Geometry: final body of the model. Coordinates: model frame, mm. A direction names the side the tool comes from. Give positions to 0.01 mm unless a question says otherwise; leave off trailing zeros. Write each loop counter-clockwise with the first axis right and the second up, starting at its lowest first coordinate (ties: lowest second). Pieces come first, ordered by that corner, then holes. Notation, with made-up numbers: (-37, -13) -> (5, -13) arc R23 ccw to (5, 22) -> close; hole circle Ø5 at (82, 71). An arc over 180 degrees is marked (long way). Answer in a Markdown table with one row per item. Add a question column.
Item 1: Material intervals for probe 1 along Y at (x, z) = (48, 13.25); probe 2 along Y at (x, z) = (31, 8.5); probe 3 along X at (y, z) = (18, 4.75), sorted ascending. Write a range as from..to.
Item 2: Section query A-A on x = 51. Output: boundary loops of the cut face in (y, z).
Item 3: Section query D-D on x = -29. Output: boundary loops of the cut face in (y, z), plus the area to 3 significant figures.
Item 4: Section query C-C on y = 31.5. Output: boundary loops of the cut face in (x, z).
Item 5: First-contact query: P1, Ø1.6, axis at x = -0.5, z = 11, coming from the +Y side. Flat tip, straight axial feed; report the tip coordinate or a pass-through.
Item 6: Access query for faces 1 (the cylindrical face through (-8.61, -38.76, 9.86)), 2 (the flat face through (-2.813, 48.08, 11.511)), 3 (the flat face through (63.72, -3.73, 12.2)). Directions: +Z, -Z, +X, -X, +Y, -Y. A direction counts if a zero-diameter tool reaches every point of the face in a straight line with its end or side. Return the directions, or none.
Item 7: Section query B-B on y = 0. Output: boundary loops of the cut face in (x, z).
Item 8: Draft query along Z for faces 4 (the cylindrical face through (-84.53, 46.98, 9.86)), 5 (the flat face through (63.72, 3.73, 7.8)), 6 (the flat face through (40, 1, 20)). Return one class per face: +Z half, -Z half, draft (parallel to the pull), parting line (faces both ways), or undercut.
```python
from build123d import *

# Parameters (mm, degrees)
SKETCH1_R               = 39.705202959
BOSS_EXTRUDE1_DEPTH     = 20
CUT_EXTRUDE1_DEPTH      = 5
CUT_EXTRUDE1_DRAFT      = -24
CUT_EXTRUDE2_REACH      = 184.868
CUT_EXTRUDE2_END_RADIUS = 39.705202959


with BuildPart() as part:
    # Sketch1 → Boss-Extrude1 (new body)
    with BuildSketch(Plane.XY):
        with BuildLine():
            Line((77.380717994, -49.989899132), (-77.380717994, -49.989899132))
            ThreePointArc((-77.380717994, -49.989899132), (-84.451785806, -47.060966943), (-87.380717994, -39.989899132))
            Line((-87.380717994, -39.989899132), (-87.380717994, 39.989899132))
            ThreePointArc((-87.380717994, 39.989899132), (-84.451785806, 47.060966943), (-77.380717994, 49.989899132))
            Line((-77.380717994, 49.989899132), (77.380717994, 49.989899132))
            ThreePointArc((77.380717994, 49.989899132), (84.451785806, 47.060966943), (87.380717994, 39.989899132))
            Line((87.380717994, 39.989899132), (87.380717994, -39.989899132))
            ThreePointArc((87.380717994, -39.989899132), (84.451785806, -47.060966943), (77.380717994, -49.989899132))
        make_face()
        Circle(SKETCH1_R, mode=Mode.SUBTRACT)
    extrude(amount=BOSS_EXTRUDE1_DEPTH)


with BuildPart() as cut_extrude1_tool:
    # Sketch2 → Cut-Extrude1 (with draft: the straight prism first)
    with BuildSketch(Plane(origin=(0, 49.989899132, 0), x_dir=(1, 0, 0), z_dir=(0, 1, 0))):
        Polygon((0, -18.082903769), (7, -5.958548116), (-7, -5.958548116), align=None)
    extrude(amount=-CUT_EXTRUDE1_DEPTH)
    # Cut-Extrude1: the draft: its side faces are tilted about the plane it starts from
    cut_extrude1_sides = [cut_extrude1_tool.faces().sort_by_distance(p)[0] for p in [
        (3.5, 47.489899132, 12.020725942),
        (0, 47.489899132, 5.958548116),
        (-3.5, 47.489899132, 12.020725942),
    ]]
    draft(cut_extrude1_sides, Plane(origin=(0, 49.989899132, 0), x_dir=(1, 0, 0), z_dir=(0, 1, 0)), CUT_EXTRUDE1_DRAFT)


with BuildPart() as part_1:
    add(part.part)

    # Cut-Extrude1: cut by cut_extrude1_tool
    add(cut_extrude1_tool.part, mode=Mode.SUBTRACT)

    # Cut-Extrude2: up to this cylinder (the profile starts outside it)
    cut_extrude2_end = Plane(origin=(0, 0, 10), z_dir=(0, 0, -1)) * Cylinder(CUT_EXTRUDE2_END_RADIUS, 450.146405919, mode=Mode.PRIVATE)
    # Sketch3 → Cut-Extrude2 (cut, up to the surface)
    with BuildSketch(Plane(origin=(87.380717994, 0, 0), x_dir=(0, 0, -1), z_dir=(1, 0, 0)), mode=Mode.PRIVATE) as cut_extrude2_sk1:
        Polygon((-10, 5), (-14.330127019, 2.5), (-14.330127019, -2.5), (-10, -5), (-5.669872981, -2.5), (-5.669872981, 2.5), align=None)
    cut_extrude2_tool1 = extrude(cut_extrude2_sk1.sketch, amount=-CUT_EXTRUDE2_REACH, mode=Mode.PRIVATE) - cut_extrude2_end
    add(cut_extrude2_tool1.solids().sort_by_distance((87.380718, 0, 10))[0], mode=Mode.SUBTRACT)


solid = part_1.part
```
Findings below:
| question | item | result |
|---|---|---|
| 1 | probe 1 | y = -49.99..-3.12, 3.12..49.99 |
| 1 | probe 2 | y = -49.99..-24.81, 24.81..49.99 |
| 1 | probe 3 | x = -87.38..-35.39, 35.39..87.38 |
| 2 | outline | (-49.99, 0) -> (49.99, 0) -> (49.99, 20) -> (-49.99, 20) -> close; hole (-5, 10) -> (-2.5, 5.67) -> (2.5, 5.67) -> (5, 10) -> (2.5, 14.33) -> (-2.5, 14.33) -> close |
| 3 | outline | (-49.99, 0) -> (-27.12, 0) -> (-27.12, 20) -> (-49.99, 20) -> close; (27.12, 0) -> (49.99, 0) -> (49.99, 20) -> (27.12, 20) -> close |
| 3 | area | 915 mm^2 |
| 4 | outline | (-87.38, 0) -> (-24.17, 0) -> (-24.17, 20) -> (-87.38, 20) -> close; (24.17, 0) -> (87.38, 0) -> (87.38, 20) -> (24.17, 20) -> close |
| 5 | P1 | stops at y = 44.99 |
| 6 | face 1 | +Z, -Z |
| 6 | face 2 | +Y |
| 6 | face 3 | +X |
| 7 | outline | (-87.38, 0) -> (-39.71, 0) -> (-39.71, 20) -> (-87.38, 20) -> close; (39.71, 0) -> (87.38, 0) -> (87.38, 5.67) -> (39.71, 5.67) -> close; (39.71, 14.33) -> (87.38, 14.33) -> (87.38, 20) -> (39.71, 20) -> close |
| 8 | face 4 | draft |
| 8 | face 5 | undercut |
| 8 | face 6 | +Z half |
